from build123d import *

# Parameters (mm, degrees)
SKETCH1_R         = 7.9375
SPACER_BOSS_DEPTH = 1.5875


with BuildPart() as part:
    # Sketch1 → Spacer Boss (new body)
    with BuildSketch(Plane.XY):
        Circle(SKETCH1_R)
        Polygon((-4.7625, 2.749630657), (-4.7625, -2.749630657), (0, -5.499261314), (4.7625, -2.749630657), (4.7625, 2.749630657), (0, 5.499261314), align=None, mode=Mode.SUBTRACT)
    extrude(amount=SPACER_BOSS_DEPTH)


solid = part.part
Can you work these out from the model? Positions are in its coordinate system, mm. A direction names the side the tool comes from. Round coordinates to 2 decimals unless told otherwise and drop trailing zeros. Loops run counter-clockwise (first coordinate to the right, second up) from the corner with the lowest first, then second, coordinate; pieces in that order, holes last. Notation, with made-up numbers: (-32.5, -39) - (-11.5, -39) arc R23 cw to (-11.5, -20) - close; hole circle Ø8 at (27.5, 44.25). An arc over 180 degrees is marked (long way). Use CSV: the item, a comma, the result in double quotes. Start each with the question number.
1) If we section it at A-A on z = 0.4: Write out the boundary of the cut face in (x, y) (1 decimal).
2) For faces 1 (the flat face through (3, 4, 0)), 2 (the flat face through (-4.762, 0, 1)), which set-ups out of +Z, -Z, +X, -X, +Y, -Y let a thin tool reach every point of the face, with its end or its side?
3) If we section it at C-C on x = -1.75: Write out the boundary of the cut face in (y, z), plus the area to 3 significant figures.
4) Please list where these lines run through material, in increasing order: probe 1 along Y at (x, z) = (2.25, 1); probe 2 along X at (y, z) = (-4, 0.75); probe 3 along X at (y, z) = (-1.75, 1.35). Write a range as [from, to].
5) We'd pull the mould along Y, two halves only. Please class faces 3 (the flat face through (2.41, 4.11, 0.78)), 4 (the cylindrical face through (-1.72, -7.75, 0.78)), 5 (the flat face through (3, 4, 1.588)): released by +Y, released by -Y, zero draft, split by the parting line, or undercut.
6) If we section it at D-D on x = 7.25: Write out the boundary of the cut face in (y, z).
7) If we section it at B-B on y = 0: Write out the boundary of the cut face in (x, z).
Geometry results:
1,outline,"circle Ø15.9 at (0, 0); hole (-4.8, -2.7) - (0, -5.5) - (4.8, -2.7) - (4.8, 2.7) - (0, 5.5) - (-4.8, 2.7) - close"
2,face 1,"-Z, +X, -X, +Y, -Y"
2,face 2,"+Z, -Z"
3,outline,"(-7.74, 0) - (-4.49, 0) - (-4.49, 1.59) - (-7.74, 1.59) - close; (4.49, 0) - (7.74, 0) - (7.74, 1.59) - (4.49, 1.59) - close"
3,area,"10.3 mm2"
4,probe 1,"y = [-7.61, -4.2], [4.2, 7.61]"
4,probe 2,"x = [-6.86, -2.6], [2.6, 6.86]"
4,probe 3,"x = [-7.74, -4.76], [4.76, 7.74]"
5,face 3,"undercut"
5,face 4,"split by the parting line"
5,face 5,"zero draft"
6,outline,"(-3.23, 0) - (3.23, 0) - (3.23, 1.59) - (-3.23, 1.59) - close"
7,outline,"(-7.94, 0) - (-4.76, 0) - (-4.76, 1.59) - (-7.94, 1.59) - close; (4.76, 0) - (7.94, 0) - (7.94, 1.59) - (4.76, 1.59) - close"
